Source: CAD feature listing. Evaluate the final solid. Frame: model axes, mm. A direction names the side the tool comes from. Round coordinates to 2 decimals unless told otherwise and drop trailing zeros. Loops run counter-clockwise (first coordinate to the right, second up) from the corner with the lowest first, then second, coordinate; pieces in that order, holes last. Notation, with made-up numbers: M 43.5,77.25 L 82.5,77.25 A35 ccw 82.5,110.25 Z; hole C 32,32.25 d3. An arc over 180 degrees is marked long. Answer as a JSON object with one key per item and string values.
from build123d import *

# Parameters (mm, degrees)
F1_DEPTH  = 20
F2_DEPTH  = 3
F0_R      = 1.7
F3_DEPTH  = 10.5
F4_R      = 1.7
F5_DEPTH  = 6.5
F6_R      = 10
F7_R      = 1.5
F8_DEPTH  = 1.5
F9_W      = 10
F9_H      = 7
F10_DEPTH = 10
F12_W     = 18.5
F12_H     = 7.2
F13_DEPTH = 2


with BuildPart() as f1:
    # F0 (on Top) → F1 (new body)
    with BuildSketch(Plane.XY):
        Polygon((-37, 31.3), (-37, -41.3), (37, -41.3), (37, 31.3), (37, 41.3), (-37, 41.3), align=None)
        Polygon((-28.8793207629, 37.1391206695), (-25.0402000934, 33.3), (25.0402000934, 33.3), (28.8793207629, 37.1391206695), (31.1655111895, 39.4253110961), (34.2885053902, 38.5885073221), (35.1253091642, 35.4655131215), (32.8391187376, 33.1793226949), (29, 29.3402039573), (29, -29.3402039573), (32.8391187376, -33.1793226949), (35.1253091642, -35.4655131215), (34.2885053902, -38.5885073221), (31.1655111895, -39.4253110961), (28.8793207629, -37.1391206695), (25.0402000934, -33.3), (-25.0402000934, -33.3), (-28.8793207629, -37.1391206695), (-31.1655111895, -39.4253110961), (-34.2885053902, -38.5885073221), (-35.1253091642, -35.4655131215), (-32.8391187376, -33.1793226949), (-29, -29.3402039573), (-29, 29.3402039573), (-32.8391187376, 33.1793226949), (-35.1253091642, 35.4655131215), (-34.2885053902, 38.5885073221), (-31.1655111895, 39.4253110961), align=None, mode=Mode.SUBTRACT)
    extrude(amount=F1_DEPTH)

    # F0 (on Top) → F2 (join)
    with BuildSketch(Plane.XY):
        Polygon((-25.0402000934, 33.3), (-29, 33.3), (-29, 29.3402039573), (-29, -29.3402039573), (-29, -33.3), (-25.0402000934, -33.3), (25.0402000934, -33.3), (29, -33.3), (29, -29.3402039573), (29, 29.3402039573), (29, 33.3), (25.0402000934, 33.3), align=None)
    extrude(amount=F2_DEPTH)

    # F0 (on Top) → F3 (join)
    with BuildSketch(Plane.XY):
        Polygon((-29, 29.3402039573), (-29, 33.3), (-25.0402000934, 33.3), (-28.8793207629, 37.1391206695), (-29.716124537, 34.0161264689), (-32.8391187376, 33.1793226949), align=None)
        Polygon((-29.716124537, 34.0161264689), (-28.8793207629, 37.1391206695), (-31.1655111895, 39.4253110961), (-34.2885053902, 38.5885073221), (-35.1253091642, 35.4655131215), (-32.8391187376, 33.1793226949), align=None)
        with Locations((-32, 36.3)):
            Circle(F0_R, mode=Mode.SUBTRACT)
        Polygon((28.8793207629, 37.1391206695), (25.0402000934, 33.3), (29, 33.3), (29, 29.3402039573), (32.8391187376, 33.1793226949), (29.716124537, 34.0161264689), align=None)
        Polygon((31.1655111895, 39.4253110961), (28.8793207629, 37.1391206695), (29.716124537, 34.0161264689), (32.8391187376, 33.1793226949), (35.1253091642, 35.4655131215), (34.2885053902, 38.5885073221), align=None)
        with Locations((32, 36.3)):
            Circle(F0_R, mode=Mode.SUBTRACT)
        Polygon((32.8391187376, -33.1793226949), (29, -29.3402039573), (29, -33.3), (25.0402000934, -33.3), (28.8793207629, -37.1391206695), (29.716124537, -34.0161264689), align=None)
        Polygon((-29, -33.3), (-29, -29.3402039573), (-32.8391187376, -33.1793226949), (-29.716124537, -34.0161264689), (-28.8793207629, -37.1391206695), (-25.0402000934, -33.3), align=None)
        Polygon((-29.716124537, -34.0161264689), (-32.8391187376, -33.1793226949), (-35.1253091642, -35.4655131215), (-34.2885053902, -38.5885073221), (-31.1655111895, -39.4253110961), (-28.8793207629, -37.1391206695), align=None)
        with Locations((-32.0023149636, -36.3023168955)):
            Circle(F0_R, mode=Mode.SUBTRACT)
        Polygon((35.1253091642, -35.4655131215), (32.8391187376, -33.1793226949), (29.716124537, -34.0161264689), (28.8793207629, -37.1391206695), (31.1655111895, -39.4253110961), (34.2885053902, -38.5885073221), align=None)
        with Locations((32, -36.3)):
            Circle(F0_R, mode=Mode.SUBTRACT)
    extrude(amount=F3_DEPTH)

    # F4 (on face) → F5 (join)
    with BuildSketch(Plane.XY.offset(20)):
        Polygon((-29, -29.3402039573), (-32.8391187376, -33.1793226949), (-29.716124537, -34.0161264689), (-28.8793207629, -37.1391206695), (-25.0402000934, -33.3), (-29, -33.3), align=None)
        Polygon((-29.716124537, -34.0161264689), (-32.8391187376, -33.1793226949), (-35.1253091642, -35.4655131215), (-34.2885053902, -38.5885073221), (-31.1655111895, -39.4253110961), (-28.8793207629, -37.1391206695), align=None)
        with Locations((-32.0023149636, -36.3023168955)):
            Circle(F4_R, mode=Mode.SUBTRACT)
        Polygon((29, -33.3), (25.0402000934, -33.3), (28.8793207629, -37.1391206695), (29.716124537, -34.0161264689), (32.8391187376, -33.1793226949), (29, -29.3402039573), align=None)
        Polygon((29.716124537, -34.0161264689), (28.8793207629, -37.1391206695), (31.1655111895, -39.4253110961), (34.2885053902, -38.5885073221), (35.1253091642, -35.4655131215), (32.8391187376, -33.1793226949), align=None)
        with Locations((32, -36.3)):
            Circle(F4_R, mode=Mode.SUBTRACT)
        Polygon((28.8793207629, 37.1391206695), (25.0402000934, 33.3), (29, 33.3), (29, 29.3402039573), (32.8391187376, 33.1793226949), (29.716124537, 34.0161264689), align=None)
        Polygon((31.1655111895, 39.4253110961), (28.8793207629, 37.1391206695), (29.716124537, 34.0161264689), (32.8391187376, 33.1793226949), (35.1253091642, 35.4655131215), (34.2885053902, 38.5885073221), align=None)
        with Locations((32, 36.3)):
            Circle(F4_R, mode=Mode.SUBTRACT)
        Polygon((-32.8391187376, 33.1793226949), (-29, 29.3402039573), (-29, 33.3), (-25.0402000934, 33.3), (-28.8793207629, 37.1391206695), (-29.716124537, 34.0161264689), align=None)
        Polygon((-35.1253091642, 35.4655131215), (-32.8391187376, 33.1793226949), (-29.716124537, 34.0161264689), (-28.8793207629, 37.1391206695), (-31.1655111895, 39.4253110961), (-34.2885053902, 38.5885073221), align=None)
        with Locations((-32, 36.3)):
            Circle(F4_R, mode=Mode.SUBTRACT)
    extrude(amount=-F5_DEPTH)

    # F6
    f6_edges = [f1.edges().sort_by_distance(p)[0] for p in [
        (29, 29.340204, 12),
        (25.0402, 33.3, 12),
        (29, -29.340204, 12),
        (25.0402, -33.3, 12),
        (-29, 29.340204, 12),
        (-25.0402, 33.3, 12),
        (-25.0402, -33.3, 12),
        (-29, -29.340204, 12),
    ]]
    fillet(f6_edges, radius=F6_R)

    # F7
    f7_edges = [f1.edges().sort_by_distance(p)[0] for p in [
        (-37, -41.3, 10),
        (37, -41.3, 10),
        (-37, 41.3, 10),
        (37, 41.3, 10),
        (-29, 33.3, 6.75),
        (-29, 33.3, 16.75),
        (29, 33.3, 6.75),
        (29, 33.3, 16.75),
        (-29, -33.3, 6.75),
        (-29, -33.3, 16.75),
        (29, -33.3, 6.75),
        (29, -33.3, 16.75),
    ]]
    fillet(f7_edges, radius=F7_R)

    # F0 (on Top) → F8 (join)
    with BuildSketch(Plane.XY):
        with Locations((32, -36.3)):
            Circle(F0_R)
        with Locations((32, 36.3)):
            Circle(F0_R)
        with Locations((-32.0023149636, -36.3023168955)):
            Circle(F0_R)
        with Locations((-32, 36.3)):
            Circle(F0_R)
    extrude(amount=F8_DEPTH)

    # F9 (on face) → F10 (cut)
    with BuildSketch(Plane(origin=(0, 41.3, 0), x_dir=(-1, 0, 0), z_dir=(0, 1, 0))):
        with Locations((0, 16.5)):
            Rectangle(F9_W, F9_H)
    extrude(amount=-F10_DEPTH, mode=Mode.SUBTRACT)

    # F12 (on face) → F13 (cut)
    with BuildSketch(Plane.XY.offset(20)):
        with Locations((-14.25, 36.9)):
            Rectangle(F12_W, F12_H)
        with Locations((14.25, 36.9)):
            Rectangle(F12_W, F12_H)
    extrude(amount=-F13_DEPTH, mode=Mode.SUBTRACT)


solid = f1.part
Item 1: Section A-A on y = -12.5. Return the cut outline in (x, z), then the cut area to 3 significant figures.
Answer sheet:
{"outline": "M -37,0 L 37,0 L 37,20 L 29,20 L 29,3 L -29,3 L -29,20 L -37,20 Z", "area": "494 mm²"}
Item 2: Section B-B on x = -1.5. Return the cut outline in (y, z), then the cut area to 3 significant figures.
Answer sheet:
{"outline": "M -41.3,0 L 41.3,0 L 41.3,13 L 33.3,13 L 33.3,3 L -33.3,3 L -33.3,20 L -41.3,20 Z", "area": "464 mm²"}
Item 3: Contact query for flat-ended pins moving along their axis: pin 1 Ø1 at (x, y) = (32.5, -36.5) entering from +Z; pin 2 Ø5.5 at (x, y) = (32, -36.3) entering from +Z; pin 3 Ø2.5 at (x, y) = (-0.5, 36) entering from +Z; pin 4 Ø3.5 at (x, y) = (17, 36.5) entering from +Z. Output: stop coordinate, or through.
Answer sheet:
{"pin 1": "stops at z = 1.5", "pin 2": "stops at z = 20", "pin 3": "stops at z = 13", "pin 4": "stops at z = 18"}
Item 4: Access query for faces 1 (the flat face through (30, 34, 13.5)), 2 (the flat face through (-32, 36, 1.5)), 3 (the flat face through (5, 37, 16)). Directions: +Z, -Z, +X, -X, +Y, -Y. A direction counts if a zero-diameter tool reaches every point of the face in a straight line with its end or side. Return the directions, or none.
Answer sheet:
{"face 1": "none", "face 2": "+Z", "face 3": "+Z, +Y"}
Item 5: Section C-C on z = 16. Return the cut outline in (x, y), then the cut area to 3 significant figures.
Answer sheet:
{"outline": "M -37,-39.8 A1.5 ccw -35.5,-41.3 L 35.5,-41.3 A1.5 ccw 37,-39.8 L 37,39.8 A1.5 ccw 35.5,41.3 L 5,41.3 L 5,33.3 L 27.5,33.3 A1.5 cw 29,31.8 L 29,-31.8 A1.5 cw 27.5,-33.3 L -27.5,-33.3 A1.5 cw -29,-31.8 L -29,31.8 A1.5 cw -27.5,33.3 L -5,33.3 L -5,41.3 L -35.5,41.3 A1.5 ccw -37,39.8 Z; hole C -32,-36.3 d3.4; hole C -32,36.3 d3.4; hole C 32,-36.3 d3.4; hole C 32,36.3 d3.4", "area": "2,130 mm²"}
Item 6: Line query: probe 1 along Y at (x, z) = (32, 6); probe 2 along X at (y, z) = (-2, 19.25); probe 3 along Y at (x, z) = (-25, 5). Output: solid intervals per line, ascending. Write a range as from..to.
Answer sheet:
{"probe 1": "y = -41.3..-38, -34.6..34.6, 38..41.3", "probe 2": "x = -37..-29, 29..37", "probe 3": "y = -41.3..-33.3, 33.3..41.3"}
Item 7: Pull-direction query (X, two-part tool) for faces 4 (the flat face through (-32.71, -39.01, 11.98)), 5 (the flat face through (0, 41.3, 10)); classes: pulls with the +X half, pulls with the -X half, needs draft (parallel to the pull), parting line crosses it, or undercut.
Answer sheet:
{"face 4": "undercut", "face 5": "needs draft"}
